Work out the finished part from the listing and answer in its coordinate system (mm). A direction names the side the tool comes from. Round coordinates to 2 decimals unless told otherwise and drop trailing zeros. Order: outer loops, then holes, each group sorted by start corner. A loop starts at its lowest first (then second) coordinate and runs counter-clockwise, first axis right, second up. Notation, with made-up numbers: (82.5, 39.5) - (118.5, 39.5) arc R10 cw to (118.5, 53.5) - close; hole circle Ø2 at (60.25, -27.5). An arc over 180 degrees is marked (long way). Put each result on its own line as item: value.
```python
from build123d import *

# Parameters (mm, degrees)
SKETCH1_W           = 150
SKETCH1_H           = 100
SKETCH1_R           = 2.55
SKETCH1_W_2         = 50
SKETCH1_H_2         = 5
BOSS_EXTRUDE1_DEPTH = 6.35
FILLET1_R           = 10


with BuildPart() as part:
    # Sketch1 → Boss-Extrude1 (new body)
    with BuildSketch(Plane(origin=(0, 0, 0), x_dir=(1, 0, 0), z_dir=(0, 1, 0))):
        Rectangle(SKETCH1_W, SKETCH1_H)
        with Locations(Location((-61, 40, 0), (0, 0, 270))):
            Circle(SKETCH1_R, mode=Mode.SUBTRACT)
        with Locations(Location((-61, 15, 0), (0, 0, 270))):
            Circle(SKETCH1_R, mode=Mode.SUBTRACT)
        with Locations((-25, 44.5)):
            Rectangle(SKETCH1_W_2, SKETCH1_H_2, mode=Mode.SUBTRACT)
        with Locations((-25, -20.5)):
            Rectangle(SKETCH1_W_2, SKETCH1_H_2, mode=Mode.SUBTRACT)
    extrude(amount=BOSS_EXTRUDE1_DEPTH)

    # Fillet1
    fillet1_edges = [part.edges().sort_by_distance(p)[0] for p in [
        (75, 3.175, 50),
        (-75, 3.175, 50),
        (-75, 3.175, -50),
        (75, 3.175, -50),
    ]]
    fillet(fillet1_edges, radius=FILLET1_R)


solid = part.part
```
1) A cutting plane is placed at A-A on z = -15. Write down the section's boundary in (x, y), then the cut area to 3 significant figures.
Findings below:
outline: (-75, 0) - (-63.55, 0) - (-63.55, 6.35) - (-75, 6.35) - close; (-58.45, 0) - (75, 0) - (75, 6.35) - (-58.45, 6.35) - close
area: 920 mm2
2) Given pin 1 Ø6 at (x, z) = (-61, -15) entering from -Y, flat-ended and moving along its own axis, determine where the tip first touches the part or whether it passes through.
Findings below:
pin 1: stops at y = 0
3) A cutting plane is placed at C-C on x = -37. Write down the section's boundary in (y, z), then the cut area to 4 significant figures.
Findings below:
outline: (0, -50) - (6.35, -50) - (6.35, -47) - (0, -47) - close; (0, -42) - (6.35, -42) - (6.35, 18) - (0, 18) - close; (0, 23) - (6.35, 23) - (6.35, 50) - (0, 50) - close
area: 571.5 mm2
4) For faces 1 (the flat face through (-50, 3, -44)), 2 (the cylindrical face through (-72.15, 3.22, 46.99)), determine the directions among +Z, -Z, +X, -X, +Y, -Y from which every point of the face is accessible in a straight line to the end or side of a thin tool.
Findings below:
face 1: +Y, -Y
face 2: +Z, -X, +Y, -Y
5) Straight lines are drawn through the part: L1, parallel to X at y = 3.5, z = -40; L2, parallel to X at y = 2, z = -41; L3, parallel to X at y = 1, z = 40.5. For each, find the intervals that lie inside material, in ascending order. Write a range as from..to.
Findings below:
L1: x = -75..-63.55, -58.45..75
L2: x = -74.95..-63.35, -58.65..74.95
L3: x = -74.99..74.99
6) For a pull along X with two mould halves and no side action, classify faces 3 (the flat face through (-25, 3, 18)), 4 (the cylindrical face through (71.99, 3.22, -47.15)), 5 (the flat face through (-1, 3, -50)) as pulls with the +X half, pulls with the -X half, needs draft (parallel to the pull), parting line crosses it, or undercut.
Findings below:
face 3: undercut
face 4: pulls with the +X half
face 5: needs draft
7) A cutting plane is placed at B-B on y = 2.75. Write down the section's boundary in (x, z).
Findings below:
outline: (-75, -40) arc R10 ccw to (-65, -50) - (65, -50) arc R10 ccw to (75, -40) - (75, 40) arc R10 ccw to (65, 50) - (-65, 50) arc R10 ccw to (-75, 40) - close; hole circle Ø5.1 at (-61, -40); hole circle Ø5.1 at (-61, -15); hole (-50, -47) - (0, -47) - (0, -42) - (-50, -42) - close; hole (-50, 18) - (0, 18) - (0, 23) - (-50, 23) - close
8) A cutting plane is placed at D-D on x = -61. Write down the section's boundary in (y, z), then the cut area to 3 significant figures.
Findings below:
outline: (0, -50) - (6.35, -50) - (6.35, -42.55) - (0, -42.55) - close; (0, -37.45) - (6.35, -37.45) - (6.35, -17.55) - (0, -17.55) - close; (0, -12.45) - (6.35, -12.45) - (6.35, 50) - (0, 50) - close
area: 570 mm2
